```python
from build123d import *

# Parameters (mm, degrees)
BOSS_EXTRUDE1_DEPTH = 33.75
SKETCH1_3_W         = 16.3
SKETCH1_3_H         = 6.6
BOSS_EXTRUDE2_DEPTH = 9.5
SKETCH2_R           = 10.975
BOSS_EXTRUDE3_DEPTH = 2.1
BOSS_EXTRUDE4_DEPTH = 19.25
SKETCH4_R           = 1.45
CUT_EXTRUDE1_DEPTH  = 4.5


with BuildPart() as part:
    # Sketch1 → Boss-Extrude1 (new body)
    with BuildSketch(Plane.XY):
        Polygon((0, 3.8), (0, 38.2), (3.8, 42), (12.7, 42), (29, 42), (38.2, 42), (42, 38.2), (42, 3.8), (38.2, 0), (3.8, 0), align=None)
    extrude(amount=BOSS_EXTRUDE1_DEPTH)

    # Sketch1_3 → Boss-Extrude2 (add)
    with BuildSketch(Plane.XY):
        with Locations((20.85, 45.3)):
            Rectangle(SKETCH1_3_W, SKETCH1_3_H)
    extrude(amount=BOSS_EXTRUDE2_DEPTH)

    # Sketch2 → Boss-Extrude3 (add)
    with BuildSketch(Plane.XY.offset(33.75)):
        with Locations((20.85, 21)):
            Circle(SKETCH2_R)
    extrude(amount=BOSS_EXTRUDE3_DEPTH)

    # Sketch3 → Boss-Extrude4 (add)
    with BuildSketch(Plane.XY.offset(35.85)):
        with BuildLine():
            Line((22.85, 22.5), (22.85, 19.5))
            ThreePointArc((22.85, 19.5), (18.35, 21), (22.85, 22.5))
        make_face()
    extrude(amount=BOSS_EXTRUDE4_DEPTH)

    # Sketch4 → Cut-Extrude1 (cut)
    with BuildSketch(Plane.XY.offset(33.75)):
        with Locations((5.5, 36.5)):
            Circle(SKETCH4_R)
        with Locations((36.5, 36.5)):
            Circle(SKETCH4_R)
        with Locations((5.5, 5.5)):
            Circle(SKETCH4_R)
        with Locations((36.5, 5.5)):
            Circle(SKETCH4_R)
    extrude(amount=-CUT_EXTRUDE1_DEPTH, mode=Mode.SUBTRACT)


solid = part.part
```
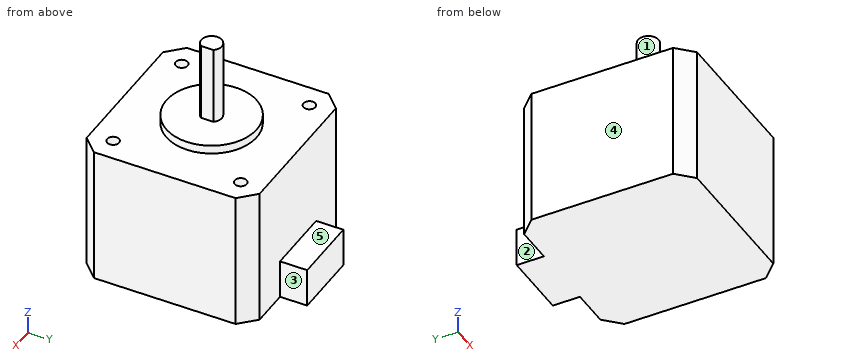
Read the model definition and answer for the solid it produces. Units are mm, in the model's axes. Face numbers are marked on the shaded views. A direction names the side the tool comes from. Give positions to 0.01 mm unless a question says otherwise; leave off trailing zeros. Write each loop counter-clockwise with the first axis right and the second up, starting at its lowest first coordinate (ties: lowest second). Pieces come first, ordered by that corner, then holes. Notation, with made-up numbers: (83, -0.75) -> (112, -0.75) arc R21 ccw to (112, 28.25) -> close; hole circle Ø9 at (0, 56). An arc over 180 degrees is marked (long way). Answer as a JSON object with one key per item and string values.
1) Section D-D on x = 13.5 is taken. Write down the section's boundary in (y, z).
Findings below:
{"outline": "(0, 0) -> (48.6, 0) -> (48.6, 9.5) -> (42, 9.5) -> (42, 33.75) -> (29.15, 33.75) -> (29.15, 35.85) -> (12.85, 35.85) -> (12.85, 33.75) -> (0, 33.75) -> close"}
2) Straight lines are drawn through the part: probe 1 along Y at (x, z) = (5.5, 31.3); probe 2 along X at (y, z) = (5, 32); probe 3 along Z at (x, y) = (19, 31). For each, find the intervals that lie inside material, in ascending order. Write a range as from..to.
Findings below:
{"probe 1": "y = 0..4.05, 6.95..35.05, 37.95..42", "probe 2": "x = 0..4.14, 6.86..35.14, 37.86..42", "probe 3": "z = 0..35.85"}
3) Flat-ended cylindrical pins translate along their axes: pin 1 Ø7.5 at (y, z) = (45.5, 5.5) entering from -X; pin 2 Ø2.5 at (x, y) = (5.5, 5.5) entering from +Z; pin 3 Ø4.5 at (x, y) = (36.5, 5.5) entering from +Z; pin 4 Ø2 at (y, z) = (34, 37) entering from -X. Find the tip coordinate at first contact, or state that the pin passes through.
Findings below:
{"pin 1": "stops at x = 3.55", "pin 2": "stops at z = 29.25", "pin 3": "stops at z = 33.75", "pin 4": "passes through"}
4) A tool of negligible diameter and unlimited length cuts with its end or side. For the marked faces 1, 2, 3, 4 and 5, from which of +Z, -Z, +X, -X, +Y, -Y can it reach the whole face along a straight path? Write none if from no direction.
Findings below:
{"face 1": "+Z", "face 2": "+Z, -Z, -X, +Y", "face 3": "+Z, -Z, +X, +Y", "face 4": "+Z, -Z, -X, +Y, -Y", "face 5": "+Z, +X, -X, +Y"}
5) Section A-A on y = 21 is taken. Write down the section's boundary in (x, z) (3 decimals), then the cut area to 3 significant figures.
Findings below:
{"outline": "(0, 0) -> (42, 0) -> (42, 33.75) -> (31.825, 33.75) -> (31.825, 35.85) -> (22.85, 35.85) -> (22.85, 55.1) -> (18.35, 55.1) -> (18.35, 35.85) -> (9.875, 35.85) -> (9.875, 33.75) -> (0, 33.75) -> close", "area": "1,550 mm^2"}
6) Section B-B on x = 5.5 is taken. Write down the section's boundary in (y, z), then the cut area to 3 significant figures.
Findings below:
{"outline": "(0, 0) -> (42, 0) -> (42, 33.75) -> (37.95, 33.75) -> (37.95, 29.25) -> (35.05, 29.25) -> (35.05, 33.75) -> (6.95, 33.75) -> (6.95, 29.25) -> (4.05, 29.25) -> (4.05, 33.75) -> (0, 33.75) -> close", "area": "1,390 mm^2"}
7) Section C-C on z = 48.5 is taken. Write down the section's boundary in (x, y).
Findings below:
{"outline": "(22.85, 19.5) -> (22.85, 22.5) arc R2.5 ccw (long way) to start"}
